Answer from the drawing. Dimensions are ordinates in mm from the lowest x, y and z of the part. Coordinates: 2 decimals unless noted, no trailing zeros. Write each loop counter-clockwise with the first axis right and the second up, starting at its lowest first coordinate (ties: lowest second). Pieces come first, ordered by that corner, then holes. Notation, with made-up numbers: (-12.5, 19.25) - (42.5, 19.25) arc R23 cw to (42.5, 47.25) - close; hole circle Ø2 at (-30.75, 89.25). An arc over 180 degrees is marked (long way). Use one line per item in the form item = value. Start each with the question number.
Item 1: A cutting plane is placed at A-A (y = 11). Write down the section's boundary in (x, z), then the cut area to 3 significant figures.
Item 2: Given pin 1 (1.6 mm diameter, centred on x = 56.5, z = 2.5, fed in from +Y); pin 2 (3 mm diameter, centred on x = 151.5, z = 1, fed in from +Y), each flat-ended and moving along its own axis, determine where each tip first touches the part or whether it passes through.
Item 3: A cutting plane is placed at C-C (x = 145). Write down the section's boundary in (y, z), then the cut area to 3 significant figures.
Item 4: Consider probe 1 along X at (y, z) = (9.25, 3.7); probe 2 along X at (y, z) = (21.75, 1.1); probe 3 along X at (y, z) = (21.5, 4.65). Determine where each line is inside the solid, lowest interval first.
Item 5: A cutting plane is placed at B-B (z = 2.8). Write down the section's boundary in (x, y), then the cut area to 3 significant figures.
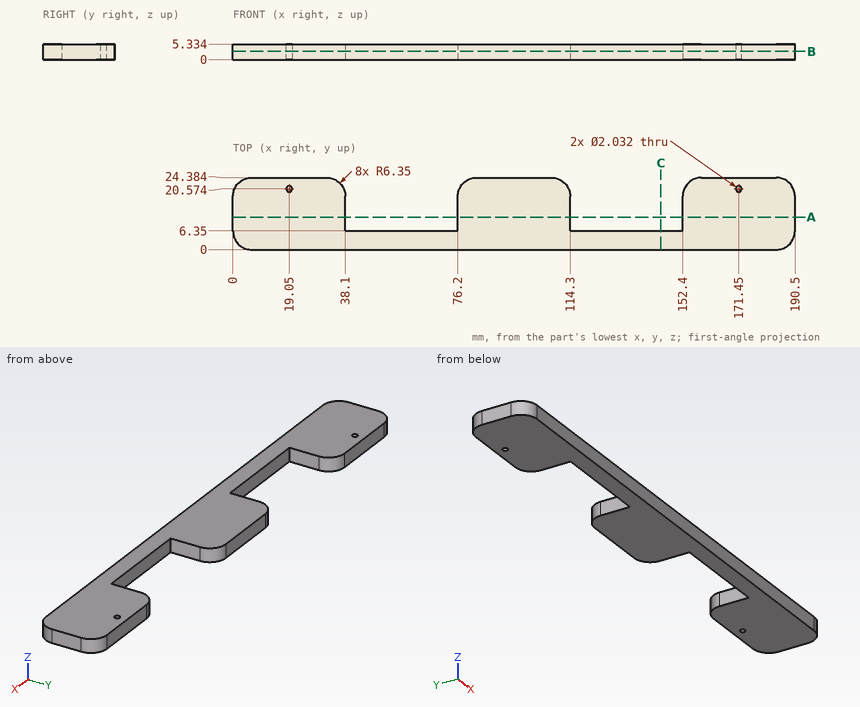
Answer:
q1.outline = (0, 0) - (38.1, 0) - (38.1, 5.33) - (0, 5.33) - close; (76.2, 0) - (114.3, 0) - (114.3, 5.33) - (76.2, 5.33) - close; (152.4, 0) - (190.5, 0) - (190.5, 5.33) - (152.4, 5.33) - close
q1.area = 610 mm²
q2.pin_1 = 6.35
q2.pin_2 = 20.73
q3.outline = (0, 0) - (6.35, 0) - (6.35, 5.33) - (0, 5.33) - close
q3.area = 33.9 mm²
q4.probe_1 = 0 to 38.1, 76.2 to 114.3, 152.4 to 190.5
q4.probe_2 = 1.2 to 36.9, 77.4 to 113.1, 153.6 to 189.3
q4.probe_3 = 1.03 to 18.63, 19.47 to 37.07, 77.23 to 113.27, 153.43 to 171.03, 171.87 to 189.47
q5.outline = (0, 6.35) arc R6.35 ccw to (6.35, 0) - (184.15, 0) arc R6.35 ccw to (190.5, 6.35) - (190.5, 18.03) arc R6.35 ccw to (184.15, 24.38) - (158.75, 24.38) arc R6.35 ccw to (152.4, 18.03) - (152.4, 6.35) - (114.3, 6.35) - (114.3, 18.03) arc R6.35 ccw to (107.95, 24.38) - (82.55, 24.38) arc R6.35 ccw to (76.2, 18.03) - (76.2, 6.35) - (38.1, 6.35) - (38.1, 18.03) arc R6.35 ccw to (31.75, 24.38) - (6.35, 24.38) arc R6.35 ccw to (0, 18.03) - close; hole circle Ø2.03 at (19.05, 20.57); hole circle Ø2.03 at (171.45, 20.57)
q5.area = 3,200 mm²
